Geometry: see drawing. Coordinates: mm, zero at the bounding-box minimum. A direction names the side the tool comes from. Round coordinates to 2 decimals unless told otherwise and drop trailing zeros. Loops run counter-clockwise (first coordinate to the right, second up) from the corner with the lowest first, then second, coordinate; pieces in that order, holes last. Notation, with made-up numbers: (70, -15) - (101, -15) arc R24 cw to (101, 3) - close; hole circle Ø10 at (60.25, -35.75). An arc over 180 degrees is marked (long way). Return JSON: item names as keys, results as strings. Group by question number.
1. Material intervals for probe 1 along Y at (x, z) = (27.5, 44.5) (1 decimal); probe 2 along X at (y, z) = (21, 9); probe 3 along X at (y, z) = (6, 44.5), sorted ascending.
2. Set-up query: the marked faces 1 and 2. Return all of +Z, -Z, +X, -X, +Y, -Y with unobstructed straight access to the full face (end or side cutting, diameter ignored); none if empty.
3. Draft query along Y for the marked faces 3, 4, 5 and 6. Return one class per face: +Y half, -Y half, draft (parallel to the pull), parting line (faces both ways), or undercut.
4. Section B-B on x = 46. Return loops of the section in (y, z) (1 decimal).
5. Section A-A on z = 16.5. Return loops of the section in (x, y) (1 decimal).
6. First-contact query: pin 1 Ø12 at (x, z) = (52.5, 37.5) entering from -Y; pin 2 Ø5 at (x, y) = (68, 3) entering from +Z; pin 3 Ø11.5 at (y, z) = (30.66, 25.4) entering from +X. Flat tips, straight axial feed; report the tip coordinate or a pass-through.
7. Section C-C on y = 51. Return loops of the section in (x, z).
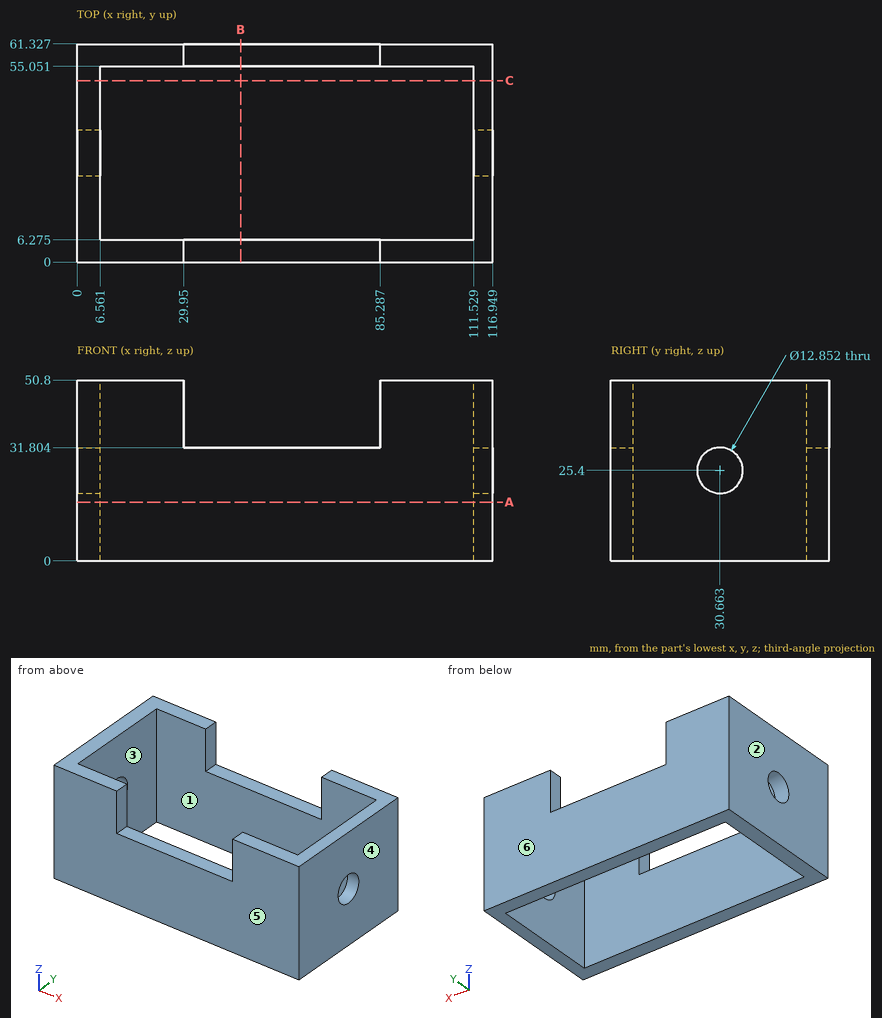
Taken from the geometry:
{
 "1": {"probe 1": "0 to 6.3, 55.1 to 61.3", "probe 2": "0 to 6.56, 111.53 to 116.95", "probe 3": "0 to 29.95, 85.29 to 116.95"},
 "2": {"face 1": "+Z, -Z", "face 2": "+Z, -Z, -X, +Y, -Y"},
 "3": {"face 3": "undercut", "face 4": "draft", "face 5": "-Y half", "face 6": "+Y half"},
 "4": {"outline": "(0, 0) - (6.3, 0) - (6.3, 31.8) - (0, 31.8) - close; (55.1, 0) - (61.3, 0) - (61.3, 31.8) - (55.1, 31.8) - close"},
 "5": {"outline": "(0, 0) - (116.9, 0) - (116.9, 61.3) - (0, 61.3) - close; hole (6.6, 6.3) - (111.5, 6.3) - (111.5, 55.1) - (6.6, 55.1) - close"},
 "6": {"pin 1": "y = 0", "pin 2": "z = 31.8", "pin 3": "through"},
 "7": {"outline": "(0, 0) - (6.56, 0) - (6.56, 50.8) - (0, 50.8) - close; (111.53, 0) - (116.95, 0) - (116.95, 50.8) - (111.53, 50.8) - close"}
}
